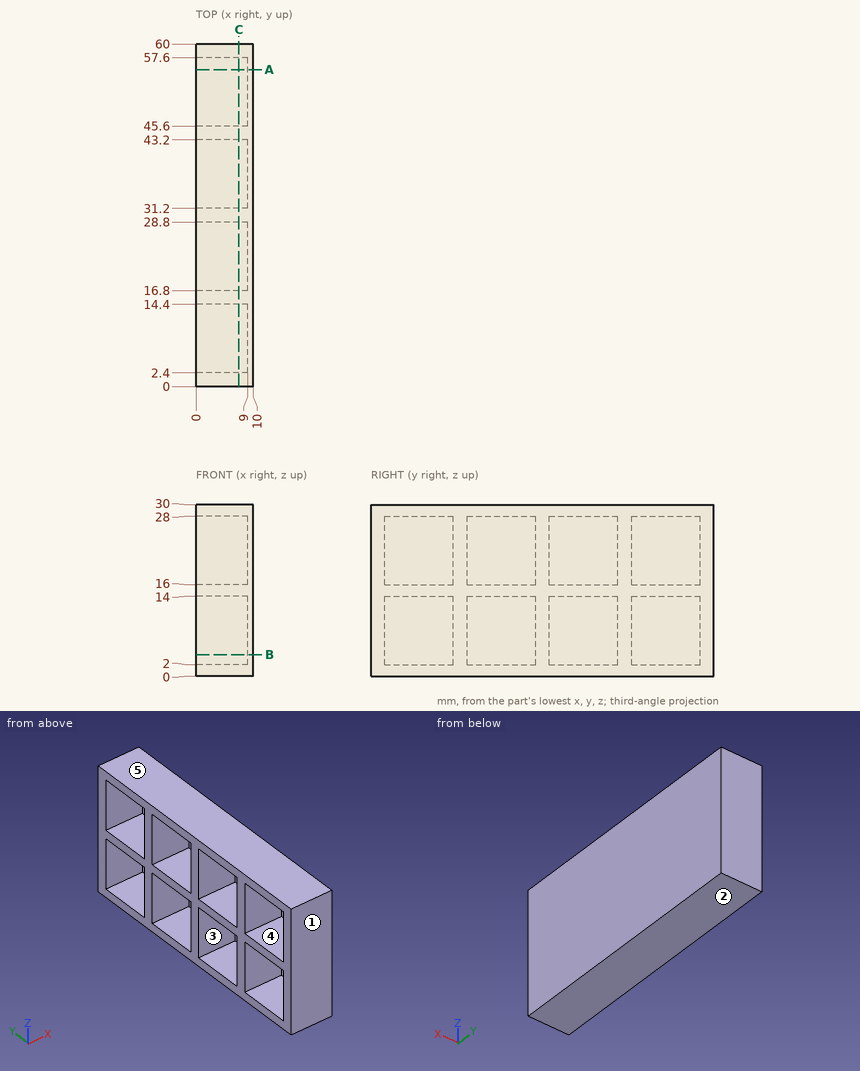
Can you work these out from the drawing? Everything is in mm from the part's minimum corner. A direction names the side the tool comes from. Give positions to 0.01 mm unless a question says otherwise; leave off trailing zeros. Order: outer loops, then holes, each group sorted by start corner. A loop starts at its lowest first (then second) coordinate and runs counter-clockwise, first axis right, second up. Notation, with made-up numbers: M 75,-17.75 L 93,-17.75 A33 ccw 93,17.25 Z; hole C 20,78.5 d6. An arc over 180 degrees is marked long. Write item = value, one per line. Start each with the question number.
Q1. Suppose I cut it at A-A (y = 55.5). Write out the boundary of the cut face in (x, z), plus the area to 3 significant figures.
Q2. Suppose I cut it at B-B (z = 3.75). Write out the boundary of the cut face in (x, y), plus the area to 3 significant figures.
Q3. Suppose I cut it at C-C (x = 7.5). Count the separate pieces of the cut face and the enclosed holes in it, plus the area to 3 significant figures.
Q4. We'd pull the mould along Y, two halves only. Please class the marked faces 1, 2 and 3: pulls with the +Y half, pulls with the -Y half, needs draft (parallel to the pull), parting line crosses it, or undercut.
Q5. For the marked faces 4 and 5, which set-ups out of +Z, -Z, +X, -X, +Y, -Y let a thin tool reach every point of the face, with its end or its side?
Q6. I need wall thicknesses on probe 1 along Y at (x, z) = (6.75, 27.25); probe 2 along Z at (x, y) = (2, 14); probe 3 along X at (y, z) = (26.5, 24.75). Which ranges of each line are inside material? Lowest first, please. Write a range as [from, to].
Q7. Will this pin go through, and if not, where does the flat tip stop? pin 1 Ø6 at (y, z) = (20.5, 10) entering from -X.
Check result:
q1.outline = M 0,0 L 10,0 L 10,30 L 0,30 L 0,28 L 9,28 L 9,16 L 0,16 L 0,14 L 9,14 L 9,2 L 0,2 Z
q1.area = 84.0 mm2
q2.outline = M 0,0 L 10,0 L 10,60 L 0,60 L 0,57.6 L 9,57.6 L 9,45.6 L 0,45.6 L 0,43.2 L 9,43.2 L 9,31.2 L 0,31.2 L 0,28.8 L 9,28.8 L 9,16.8 L 0,16.8 L 0,14.4 L 9,14.4 L 9,2.4 L 0,2.4 Z
q2.area = 168 mm2
q3.separate_pieces = 1
q3.enclosed_holes = 8
q3.area = 648 mm2
q4.face_1 = pulls with the -Y half
q4.face_2 = needs draft
q4.face_3 = undercut
q5.face_4 = -X
q5.face_5 = +Z, +X, -X, +Y, -Y
q6.probe_1 = [0, 2.4], [14.4, 16.8], [28.8, 31.2], [43.2, 45.6], [57.6, 60]
q6.probe_2 = [0, 2], [14, 16], [28, 30]
q6.probe_3 = [9, 10]
q7.pin_1 = 9
